Autodesk Inventor part; units mm, degrees
ref_plane "YZ Plane" through (0, 0, 0) normal (1, 0, 0) x (0, 1, 0)
ref_plane "XZ Plane" through (0, 0, 0) normal (0, 1, 0) x (-1, 0, 0)
ref_plane "XY Plane" through (0, 0, 0) normal (0, 0, 1) x (1, 0, 0)
sketch "Sketch1" plane through (0, 0, 0) normal (1, 0, 0) x (0, 1, 0)
  line L0 (119.0767, 81.9121) -> (-121.9233, 81.9121)
  line L1 (-121.9233, 81.9121) -> (-121.9233, -0.0879)
  line L2 (-121.9233, -0.0879) -> (119.0767, -0.0879)
  line L3 (119.0767, -0.0879) -> (119.0767, 81.9121)
  circle A0 centre (-54.9233, 40.9121) radius 19
  line L4 (-121.9233, 73.9121) -> (-118.9233, 73.9121)
  line L5 (-118.9233, 73.9121) -> (-118.9233, 7.9121)
  line L6 (-118.9233, 7.9121) -> (-121.9233, 7.9121)
  line L7 (-121.9233, 7.9121) -> (-121.9233, 73.9121)
  circle A1 centre (26.2941, 56.2319) radius 2.35
  circle A2 centre (16.2941, 56.2319) radius 2.35
  circle A3 centre (6.2941, 56.2319) radius 2.35
  circle A4 centre (-3.7059, 56.2319) radius 2.35
  circle A5 centre (-13.7059, 56.2319) radius 2.35
  circle A6 centre (26.2941, 46.2319) radius 2.35
  circle A7 centre (16.2941, 46.2319) radius 2.35
  circle A8 centre (6.2941, 46.2319) radius 2.35
  circle A9 centre (-3.7059, 46.2319) radius 2.35
  circle A10 centre (-13.7059, 46.2319) radius 2.35
  circle A11 centre (26.2941, 36.2319) radius 2.35
  circle A12 centre (16.2941, 36.2319) radius 2.35
  circle A13 centre (6.2941, 36.2319) radius 2.35
  circle A14 centre (-3.7059, 36.2319) radius 2.35
  circle A15 centre (-13.7059, 36.2319) radius 2.35
  circle A16 centre (26.2941, 26.2319) radius 2.35
  circle A17 centre (16.2941, 26.2319) radius 2.35
  circle A18 centre (6.2941, 26.2319) radius 2.35
  circle A19 centre (-3.7059, 26.2319) radius 2.35
  circle A20 centre (-13.7059, 26.2319) radius 2.35
  point P0 (0, 0)
  point P1 (0, 0)
  dimension "d0" = 241
  dimension "d1" = 82
  dimension "d2" = 38
  dimension "d3" = 41
  dimension "d4" = 174
  dimension "d5" = 66
  dimension "d6" = 3
  dimension "d7" = 8
  dimension "d21" = 4.7
  dimension "d24" = 10
  dimension "d27" = 10
extrude "Extrusion1" add sketch "Sketch1" along normal blind 5 contours L3 L2 L1 L6 L5 L4 L0 | A0
equation "\"d3\" = 0.5 * d1"
equation "\"d7\" = -0.5 * d5 + 0.5 * d1"
properties part number "inner_2Poke"
Geometry: final body of the model. Coordinates: model frame, mm. A direction names the side the tool comes from. Round coordinates to 2 decimals unless told otherwise and drop trailing zeros. Write item = value, one per line.
Item 1: Section query A-A on x = 1.75. State how many separate pieces and enclosed holes the cut face has, then the cut area to 3 significant figures.
Findings:
separate_pieces = 1
enclosed_holes = 20
area = 19,200 mm^2
Item 2: Pin query (flat end, axial travel): P1, Ø3, axis at y = -13.71, z = 26.23, coming from the +X side; P2, Ø3, axis at x = 1.5, z = 30, coming from the -Y side. Return the tip coordinate at first contact, or that it passes through.
Findings:
P1 = through
P2 = -118.92
Item 3: Access query for faces 1 (the face through (2, -118.923, 41)), 2 (the face through (2.465, 27.378, 58.317)). Directions: +Z, -Z, +X, -X, +Y, -Y. A direction counts if a zero-diameter tool reaches every point of the face in a straight line with its end or side. Return the directions, or none.
Findings:
face_1 = +X, -X, -Y
face_2 = +X, -X
Item 4: Material intervals for line 1 along Y through (x, z) = (2.1, 45.5); line 2 along Z through (x, y) = (2.2, -3); line 3 along Y through (x, z) = (0.45, 27.5), sorted ascending. Write a range as [from, to].
Findings:
line_1 = [-118.92, -15.94], [-11.47, -5.94], [-1.47, 4.06], [8.53, 14.06], [18.53, 24.06], [28.53, 119.08]
line_2 = [-0.09, 23.99], [28.47, 33.99], [38.47, 43.99], [48.47, 53.99], [58.47, 81.91]
line_3 = [-118.92, -15.68], [-11.73, -5.68], [-1.73, 4.32], [8.27, 14.32], [18.27, 24.32], [28.27, 119.08]
Item 5: Pull-direction query (Y, two-part tool) for faces 3 (the face through (2, 0, 81.912)), 4 (the face through (2.465, 5.785, 28.526)), 5 (the face through (2, 119.077, 40)); classes: pulls with the +Y half, pulls with the -Y half, needs draft (parallel to the pull), parting line crosses it, or undercut.
Findings:
face_3 = needs draft
face_4 = undercut
face_5 = pulls with the +Y half
